Here's how the part is built. I have some questions about the finished solid (model axes, mm). A direction names the side the tool comes from. Coordinates: 2 decimals unless noted, no trailing zeros. Write each loop counter-clockwise with the first axis right and the second up, starting at its lowest first coordinate (ties: lowest second). Pieces come first, ordered by that corner, then holes. Notation, with made-up numbers: (53.25, 21) -> (75.25, 21) arc R16 ccw to (75.25, 45) -> close; hole circle Ø5 at (45.5, 4). An arc over 180 degrees is marked (long way). Put each result on its own line as item: value. Start each with the question number.
Item 1: I need wall thicknesses on line 1 (Z direction, x = 0, y = 7.05); line 2 (Z direction, x = 0, y = -6.9); line 3 (X direction, y = -5.25, z = 219). Which ranges of each line are inside material? Lowest first, please. Write a range as [from, to].
Item 2: If we mould it in two halves opening along X, with no side actions, what happens to faces 4 (the face through (-7, 0, 300)), 5 (the face through (7.5, 0, 148)), 6 (the face through (-0.651, 6.76, 2.543))? For each: released by +X, released by -X, zero draft, split by the parting line, or undercut.
Item 3: For pin 1 (5 mm diameter, centred on x = 0, z = 262.5, fed in from +Y), with a flat end and sliding along its axis, tell me the tip position at first contact or that it passes through.
Item 4: On a 3-axis mill with a long thin cutter (end or side, diameter ignored), from which of +Z, -Z, +X, -X, +Y, -Y can I reach the whole of each face in a straight line? I mean faces 1 (the face through (-6, 0, 148)), 2 (the face through (0, -7.5, 148)), 3 (the face through (-0.651, 6.76, 287.543)). Say none if no direction works.
Item 5: I want a section at A-A, the plane y = -2.75. List the corners of the cut face in (x, z) for me.
Item 6: I want a section at B-B, the plane z = 24. List the corners of the cut face in (x, y) for me.
from build123d import *

# Parameters (mm, degrees)
SKETCH_1_W          = 15
SKETCH_1_H          = 15
SKETCH_1_W_2        = 12
SKETCH_1_H_2        = 12
EXTRUDE_1_DEPTH     = 300
SKETCH_5_R          = 2
CUT_EXTRUDE_4_DEPTH = 20
SKETCH_8_R          = 5
CUT_EXTRUDE_5_DEPTH = 10


with BuildPart() as part:
    # ｽｹｯﾁ1 → ﾎﾞｽ - 押し出し1 (new body)
    with BuildSketch(Plane.XY):
        Rectangle(SKETCH_1_W, SKETCH_1_H)
        Rectangle(SKETCH_1_W_2, SKETCH_1_H_2, mode=Mode.SUBTRACT)
    extrude(amount=EXTRUDE_1_DEPTH)

    # ｽｹｯﾁ5 → ｶｯﾄ - 押し出し4 (cut)
    with BuildSketch(Plane(origin=(0, -7.5, 0), x_dir=(-1, 0, 0), z_dir=(0, -1, 0))):
        with Locations((0, -37.5)):
            Circle(SKETCH_5_R)
        with Locations((0, -7.5)):
            Circle(SKETCH_5_R)
        with Locations((0, -292.5)):
            Circle(SKETCH_5_R)
        with Locations((0, -262.5)):
            Circle(SKETCH_5_R)
    extrude(amount=-CUT_EXTRUDE_4_DEPTH, mode=Mode.SUBTRACT)

    # ｽｹｯﾁ8 → ｶｯﾄ - 押し出し5 (cut)
    with BuildSketch(Plane(origin=(0, 7.5, 0), x_dir=(1, 0, 0), z_dir=(0, 1, 0))):
        with Locations((0, -292.5)):
            Circle(SKETCH_8_R)
        with Locations((0, -262.5)):
            Circle(SKETCH_8_R)
        with Locations((0, -37.5)):
            Circle(SKETCH_8_R)
        with Locations((0, -7.5)):
            Circle(SKETCH_8_R)
    extrude(amount=-CUT_EXTRUDE_5_DEPTH, mode=Mode.SUBTRACT)


solid = part.part
Calculated:
1. line 1: z = [0, 2.5], [12.5, 32.5], [42.5, 257.5], [267.5, 287.5], [297.5, 300]
1. line 2: z = [0, 5.5], [9.5, 35.5], [39.5, 260.5], [264.5, 290.5], [294.5, 300]
1. line 3: x = [-7.5, -6], [6, 7.5]
2. face 4: zero draft
2. face 5: released by +X
2. face 6: undercut
3. pin 1: stops at y = -6
4. face 1: +Z, -Z
4. face 2: +Z, -Z, +X, -X, -Y
4. face 3: +Y
5. outline: (-7.5, 0) -> (-6, 0) -> (-6, 300) -> (-7.5, 300) -> close; (6, 0) -> (7.5, 0) -> (7.5, 300) -> (6, 300) -> close
6. outline: (-7.5, -7.5) -> (7.5, -7.5) -> (7.5, 7.5) -> (-7.5, 7.5) -> close; hole (-6, -6) -> (6, -6) -> (6, 6) -> (-6, 6) -> close
